from build123d import *

# Parameters (mm, degrees)
SKETCH_1_W           = 43
SKETCH_1_H           = 38
EXTRUDE_1_DEPTH      = 9
SKETCH_2_W           = 43
SKETCH_2_H           = 3
EXTRUDE_3_DEPTH      = 51
SKETCH_3_R           = 1.900733336
CUT_EXTRUDE_1_DEPTH  = 42
SKETCH_4_W           = 5
SKETCH_4_H           = 6
CUT_EXTRUDE_2_DEPTH  = 44
SKETCH_8_R           = 1.25
CUT_EXTRUDE_6_DEPTH  = 9
SKETCH_7_R           = 1.2
CUT_EXTRUDE_7_DEPTH  = 15
SKETCH_9_W           = 10.2
SKETCH_9_H           = 13
CUT_EXTRUDE_8_DEPTH  = 1.3
SKETCH_11_W          = 7
SKETCH_11_H          = 12.5
CUT_EXTRUDE_13_DEPTH = 3.7
SKETCH_10_R          = 1.25
CUT_EXTRUDE_14_DEPTH = 8
FILLET_1_R           = 1
FILLET_2_R           = 1


with BuildPart() as part:
    # Эскиз1 → Бобышка-Вытянуть1 (new body)
    with BuildSketch(Plane.XY):
        Rectangle(SKETCH_1_W, SKETCH_1_H)
    extrude(amount=EXTRUDE_1_DEPTH)

    # Эскиз2 → Бобышка-Вытянуть3 (add)
    with BuildSketch(Plane.XY.offset(9)):
        with Locations((0, -20.5)):
            Rectangle(SKETCH_2_W, SKETCH_2_H)
    extrude(amount=-EXTRUDE_3_DEPTH)

    # Эскиз3 → Вырез-Вытянуть1 (cut, through all)
    with BuildSketch(Plane.XZ.offset(22)):
        with Locations(Location((-13, -38.5, 0), (0, 0, 270))):  # turned: the seam where the file's is
            Circle(SKETCH_3_R)
        with Locations(Location((13, -38.5, 0), (0, 0, 270))):  # turned: the seam where the file's is
            Circle(SKETCH_3_R)
        with Locations(Location((13, -13.5, 0), (0, 0, 270))):  # turned: the seam where the file's is
            Circle(SKETCH_3_R)
        with Locations(Location((-13, -13.5, 0), (0, 0, 270))):  # turned: the seam where the file's is
            Circle(SKETCH_3_R)
    extrude(amount=-CUT_EXTRUDE_1_DEPTH, mode=Mode.SUBTRACT)

    # Эскиз4 → Вырез-Вытянуть2 (cut, through all)
    with BuildSketch(Plane.ZY.offset(21.5)):
        with Locations((2.5, 16)):
            Rectangle(SKETCH_4_W, SKETCH_4_H)
    extrude(amount=-CUT_EXTRUDE_2_DEPTH, mode=Mode.SUBTRACT)

    # Эскиз8 → Вырез-Вытянуть6 (cut)
    with BuildSketch(Plane.XY.offset(9)):
        with Locations((16.5, -17)):
            Circle(SKETCH_8_R)
        with Locations((-16.5, -17)):
            Circle(SKETCH_8_R)
    extrude(amount=-CUT_EXTRUDE_6_DEPTH, mode=Mode.SUBTRACT)

    # Эскиз7 → Вырез-Вытянуть7 (cut)
    with BuildSketch(Plane(origin=(0, 13, 0), x_dir=(1, 0, 0), z_dir=(0, 1, 0))):
        with Locations(Location((16.5, -2.5, 0), (0, 0, 270))):  # turned: the seam where the file's is
            Circle(SKETCH_7_R)
        with Locations(Location((6.5, -2.5, 0), (0, 0, 270))):  # turned: the seam where the file's is
            Circle(SKETCH_7_R)
        with Locations(Location((-3.5, -2.5, 0), (0, 0, 270))):  # turned: the seam where the file's is
            Circle(SKETCH_7_R)
    extrude(amount=-CUT_EXTRUDE_7_DEPTH, mode=Mode.SUBTRACT)

    # Эскиз9 → Вырез-Вытянуть8 (cut)
    with BuildSketch(Plane.XY.offset(9)):
        with Locations((-13.15, 12.5)):
            Rectangle(SKETCH_9_W, SKETCH_9_H)
    extrude(amount=-CUT_EXTRUDE_8_DEPTH, mode=Mode.SUBTRACT)

    # Эскиз11 → Вырез-Вытянуть13 (cut)
    with BuildSketch(Plane.XY.offset(7.7)):
        with Locations((-13.15, 12.75)):
            Rectangle(SKETCH_11_W, SKETCH_11_H)
    extrude(amount=-CUT_EXTRUDE_13_DEPTH, mode=Mode.SUBTRACT)

    # Эскиз10 → Вырез-Вытянуть14 (cut)
    with BuildSketch(Plane.XY.offset(7.7)):
        with Locations((-13.149995044, 9.4)):
            Circle(SKETCH_10_R)
    extrude(amount=-CUT_EXTRUDE_14_DEPTH, mode=Mode.SUBTRACT)

    # Скругление1
    fillet_1_edges = [part.edges().sort_by_distance(p)[0] for p in [
        (-16.65, 6.5, 5.85),
        (-9.65, 6.5, 5.85),
    ]]
    fillet(fillet_1_edges, radius=FILLET_1_R)

    # Скругление2
    fillet_2_edges = [part.edges().sort_by_distance(p)[0] for p in [
        (-8.05, 6, 8.35),
        (-18.25, 6, 8.35),
    ]]
    fillet(fillet_2_edges, radius=FILLET_2_R)


solid = part.part
The model under review builds one solid part; all positions refer to its coordinate system, in mm. A direction names the side the tool comes from. Coordinates: 2 decimals unless noted, no trailing zeros. Write each loop counter-clockwise with the first axis right and the second up, starting at its lowest first coordinate (ties: lowest second). Pieces come first, ordered by that corner, then holes. Notation, with made-up numbers: (22, 72) - (54, 72) arc R35 cw to (54, 107) - close; hole circle Ø7 at (-3, 44). An arc over 180 degrees is marked (long way). Answer as a JSON object with one key per item and string values. Group by question number.
1. Add section D-D (x = -3.5). Give the boundary of the cut face in (y, z), plus the area to 3 significant figures.
2. Add section A-A (y = 15.5). Give the boundary of the cut face in (x, z).
3. Add section B-B (z = -13.5). Give the boundary of the cut face in (x, y).
4. Clearance check with flat-ended pins moving along their axes: pin 1 Ø5 at (x, y) = (-12.5, 10.5) entering from -Z; pin 2 Ø1.8 at (x, y) = (10.5, 14.5) entering from -Z; pin 3 Ø2 at (x, z) = (6.5, 2.5) entering from +Y. State where each tip first meets the part, or that it passes through.
5. Machinability: for faces 4 (the face through (-13.728, -20.521, -40.256)), 5 (the face through (-13, 6.5, 6)), 6 (the face through (0, -3, 0)), which of the approach directions +Z, -Z, +X, -X, +Y, -Y give a long, thin tool a straight path to every point of the face, cutting with its end or side? Answer none if there is none.
6. Add section C-C (x = 16.5). Give the boundary of the cut face in (y, z), plus the area to 4 significant figures.
7. Mouldability with a two-part tool opening along Z and no side actions: class faces 1 (the face through (0, -20, -42)), 2 (the face through (12.272, -20.521, -40.256)), 3 (the face through (-18.25, 13, 8)) as pulls with the +Z half, pulls with the -Z half, needs draft (parallel to the pull), parting line crosses it, or undercut.
8. To check wall thickness, follow probe 1 along X at (y, z) = (-20.9, -38.5); probe 2 along X at (y, z) = (4, 2.5); probe 3 along X at (y, z) = (9.75, 2.5). State the ranges of each line that lie inside material, in increasing order.
Findings:
{
 "1": {"outline": "(-22, -42) - (-19, -42) - (-19, 0) - (13, 0) - (13, 1.3) - (-2, 1.3) - (-2, 3.7) - (13, 3.7) - (13, 5) - (19, 5) - (19, 9) - (-22, 9) - close", "area": "429 mm²"},
 "2": {"outline": "(-21.5, 5) - (-16.65, 5) - (-16.65, 7.7) - (-18.25, 7.7) - (-18.25, 9) - (-21.5, 9) - close; (-9.65, 5) - (21.5, 5) - (21.5, 9) - (-8.05, 9) - (-8.05, 7.7) - (-9.65, 7.7) - close"},
 "3": {"outline": "(-21.5, -22) - (-14.9, -22) - (-14.9, -19) - (-21.5, -19) - close; (-11.1, -22) - (11.1, -22) - (11.1, -19) - (-11.1, -19) - close; (14.9, -22) - (21.5, -22) - (21.5, -19) - (14.9, -19) - close"},
 "4": {"pin 1": "z = 0", "pin 2": "z = 5", "pin 3": "y = -2"},
 "5": {"face 4": "+Y, -Y", "face 5": "+Z, +Y", "face 6": "-Z, +X, -X, +Y"},
 "6": {"outline": "(-22, -42) - (-19, -42) - (-19, 0) - (-18.25, 0) - (-18.25, 9) - (-22, 9) - close; (-15.75, 0) - (13, 0) - (13, 1.3) - (-2, 1.3) - (-2, 3.7) - (13, 3.7) - (13, 5) - (19, 5) - (19, 9) - (-15.75, 9) - close", "area": "406.5 mm²"},
 "7": {"face 1": "pulls with the -Z half", "face 2": "undercut", "face 3": "needs draft"},
 "8": {"probe 1": "-21.5 to -14.9, -11.1 to 11.1, 14.9 to 21.5", "probe 2": "-21.5 to -4.7, -2.3 to 5.3, 7.7 to 15.3, 17.7 to 21.5", "probe 3": "-21.5 to -14.35, -11.95 to -4.7, -2.3 to 5.3, 7.7 to 15.3, 17.7 to 21.5"}
}
